```python
from build123d import *

# Parameters (mm, degrees)
SKETCH1_R           = 23
BOSS_EXTRUDE1_DEPTH = 3
SKETCH2_R           = 1.5
CUT_EXTRUDE1_DEPTH  = 10
SKETCH3_R           = 5
CUT_EXTRUDE2_DEPTH  = 10
CUT_EXTRUDE3_DEPTH  = 10
FILLET1_R           = 1


with BuildPart() as part:
    # Sketch1 → Boss-Extrude1 (new body)
    with BuildSketch(Plane(origin=(0, 0, 0), x_dir=(1, 0, 0), z_dir=(0, 1, 0))):
        with Locations(Location((0, 0, 0), (0, 0, 270))):
            Circle(SKETCH1_R)
    extrude(amount=BOSS_EXTRUDE1_DEPTH)

    # Sketch2 → Cut-Extrude1 (cut)
    with BuildSketch(Plane.XZ):
        with Locations(Location((-12.45, 3, 0), (0, 0, 270))):
            Circle(SKETCH2_R)
        with Locations(Location((10.5, -3, 0), (0, 0, 270))):
            Circle(SKETCH2_R)
    extrude(amount=-CUT_EXTRUDE1_DEPTH, mode=Mode.SUBTRACT)

    # Sketch3 → Cut-Extrude2 (cut)
    with BuildSketch(Plane(origin=(0, 3, 0), x_dir=(1, 0, 0), z_dir=(0, 1, 0))):
        with Locations(Location((0, 0, 0), (0, 0, 270))):
            Circle(SKETCH3_R)
    extrude(amount=-CUT_EXTRUDE2_DEPTH, mode=Mode.SUBTRACT)

    # Sketch4 → Cut-Extrude3 (cut)
    with BuildSketch(Plane(origin=(0, 3, 0), x_dir=(1, 0, 0), z_dir=(0, 1, 0))):
        Polygon((-4.999542106, 0.067666304), (-4.999542106, -6.72215), (-4.999542106, -11.432488216), (-23.949207952, -11.432488216), (-23.949207952, -24.872488216), (-5.202998913, -24.872488216), (4.797001087, -24.872488216), (29.316778345, -24.872488216), (29.316778345, -11.432488216), (4.999542106, -11.432488216), (4.999542106, 0.067666304), align=None)
    extrude(amount=-CUT_EXTRUDE3_DEPTH, mode=Mode.SUBTRACT)

    # Fillet1
    fillet1_edges = [part.edges().sort_by_distance(p)[0] for p in [
        (19.957409982, 1.5, 11.432488216),
        (4.999542106, 1.5, 11.432488216),
        (-19.957409982, 1.5, 11.432488216),
        (-4.999542106, 1.5, 11.432488216),
    ]]
    fillet(fillet1_edges, radius=FILLET1_R)


solid = part.part
```
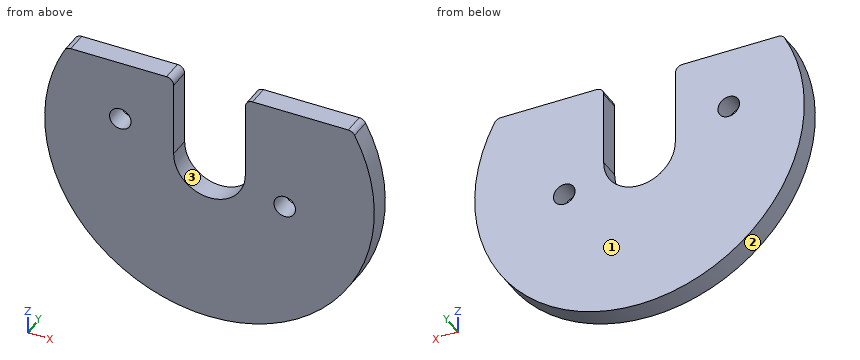
Check sheet for the modelled part. Datum: model origin and axes. Units: mm. Face numbers are marked on the shaded views. Coordinates: 2 decimals unless noted, no trailing zeros. Loops run counter-clockwise (first coordinate to the right, second up) from the corner with the lowest first, then second, coordinate; pieces in that order, holes last. Notation, with made-up numbers: M 2.5,-27 L 20.5,-27 A19 cw 20.5,-14 Z; hole C 21,11 d8. An arc over 180 degrees is marked long. Answer as a JSON object with one key per item and string values.
1. Sectioned sample at B-B on z = 3.5. Record the cut outline in (x, y).
Outcome:
{"outline": "M -22.73,0 L -13.86,0 L -13.86,3 L -22.73,3 Z; M -11.04,0 L -5,0 L -5,3 L -11.04,3 Z; M 5,0 L 22.73,0 L 22.73,3 L 5,3 Z"}
2. Depth check by flat-ended pin: P1, Ø0.9, axis at y = 1, z = 5, coming from the -X side; P2, Ø1.8, axis at x = -12.45, z = 3, coming from the +Y side; P3, Ø0.9, axis at y = 2, z = 5.5, coming from the +X side. Enter the tip coordinate at first touch or a pass-through.
Outcome:
{"P1": "x = -22.55", "P2": "through", "P3": "x = 22.44"}
3. Sectioned sample at D-D on z = -3. Record the cut outline in (x, y), and give its area (3 significant figures).
Outcome:
{"outline": "M -22.8,0 L -4,0 L -4,3 L -22.8,3 Z; M 4,0 L 9,0 L 9,3 L 4,3 Z; M 12,0 L 22.8,0 L 22.8,3 L 12,3 Z", "area": "104 mm²"}
4. Release check for a two-part mould opening along X. For the marked faces 1, 2 and 3 record: pulls with the +X half, pulls with the -X half, needs draft (parallel to the pull), parting line crosses it, or undercut.
Outcome:
{"face 1": "needs draft", "face 2": "parting line crosses it", "face 3": "undercut"}
5. Scan lines: L1, parallel to X at y = 0.25, z = -2.5; L2, parallel to X at y = 1.6, z = 3; L3, parallel to X at y = 0.15, z = 9. Record each from-to range of solid material in increasing order. Write a range as from..to.
Outcome:
{"L1": "-22.86..-4.33, 4.33..9.09, 11.91..22.86", "L2": "-22.8..-13.95, -10.95..-5, 5..22.8", "L3": "-21.17..-5, 5..21.17"}
6. Sectioned sample at C-C on x = -12.45. Record the cut outline in (y, z), and give its area (3 significant figures).
Outcome:
{"outline": "M 0,-19.34 L 3,-19.34 L 3,1.5 L 0,1.5 Z; M 0,4.5 L 3,4.5 L 3,11.43 L 0,11.43 Z", "area": "83.3 mm²"}
7. Sectioned sample at A-A on y = 1.05. Record the cut outline in (x, z).
Outcome:
{"outline": "M -20.25,10.91 A23 ccw long 20.25,10.91 A1 ccw 19.37,11.43 L 6,11.43 A1 ccw 5,10.43 L 5,0.07 A5 cw long -5,0.07 L -5,10.43 A1 ccw -6,11.43 L -19.37,11.43 A1 ccw Z; hole C -12.45,3 d3; hole C 10.5,-3 d3"}
